Part model, mm, in its own coordinate system. A direction names the side the tool comes from. Round coordinates to 2 decimals unless told otherwise and drop trailing zeros.
```python
from build123d import *

# Parameters (mm, degrees)
SKETCH1_R           = 42.5
BOSS_EXTRUDE1_DEPTH = 115
SKETCH2_R           = 41
CUT_EXTRUDE3_DEPTH  = 115
SKETCH9_W           = 4.5
SKETCH9_H           = 9
CUT_EXTRUDE5_DEPTH  = 115
SKETCH14_W          = 4
SKETCH14_H          = 2.5
CUT_EXTRUDE8_DEPTH  = 115
SKETCH16_W          = 8
SKETCH16_H          = 4.5
CUT_EXTRUDE9_DEPTH  = 115
BOSS_EXTRUDE2_START = 1
SKETCH19_R          = 41
BOSS_EXTRUDE2_DEPTH = 1
SKETCH21_R          = 3
BOSS_EXTRUDE3_DEPTH = 50
SHELL1_T            = -0.3
SKETCH24_R          = 3
BOSS_EXTRUDE4_DEPTH = 35
SHELL2_START        = 19
SHELL2_OUTLINE_R    = 2.7
SHELL2_DEPTH        = 35
SKETCH25_R          = 3
BOSS_EXTRUDE5_DEPTH = 45
SHELL5_T            = -0.03
SKETCH26_W          = 30
SKETCH26_H          = 15
BOSS_EXTRUDE6_DEPTH = 5


# Read off the part's stored shape, not the designer's step: Shell2
with BuildPart() as part:
    # Sketch1 → Boss-Extrude1 (new body)
    with BuildSketch(Plane(origin=(0, 0, 0), x_dir=(1, 0, 0), z_dir=(0, 1, 0))):
        with Locations(Location((0, 0, 0), (0, 0, 270))):
            Circle(SKETCH1_R)
    extrude(amount=BOSS_EXTRUDE1_DEPTH)

    # Sketch7 → Loft2 section 0
    with BuildSketch(Plane.XZ):
        with BuildLine():
            Line((-15.1377027, -38.271634302), (14.891561193, -38.271634302))
            Line((14.891561193, -38.271634302), (14.891561193, -51.96970786))
            Line((14.891561193, -51.96970786), (-15.1377027, -51.96970786))
            Line((-15.1377027, -51.96970786), (-15.1377027, -38.271634302))
        make_face()
    # Sketch6 → Loft2 section 1
    with BuildSketch(Plane(origin=(0, 115, 0), x_dir=(1, 0, 0), z_dir=(0, 1, 0))):
        with BuildLine():
            Line((-10.741203576, 39.96970786), (9.258796424, 39.96970786))
            Line((9.258796424, 39.96970786), (9.258796424, 51.96970786))
            Line((9.258796424, 51.96970786), (-10.741203576, 51.96970786))
            Line((-10.741203576, 51.96970786), (-10.741203576, 39.96970786))
        make_face()
    loft()

    # Sketch2 → Cut-Extrude3 (cut)
    with BuildSketch(Plane(origin=(0, 115, 0), x_dir=(1, 0, 0), z_dir=(0, 1, 0))):
        with Locations(Location((0, 0, 0), (0, 0, 270))):
            Circle(SKETCH2_R)
    extrude(amount=-CUT_EXTRUDE3_DEPTH, mode=Mode.SUBTRACT)

    # Sketch9 → Cut-Extrude5 (cut)
    with BuildSketch(Plane(origin=(0, 115, 0), x_dir=(1, 0, 0), z_dir=(0, 1, 0))):
        with Locations((-6.991203576, 47.46970786)):
            Rectangle(SKETCH9_W, SKETCH9_H)
        with Locations((5.508796424, 47.46970786)):
            Rectangle(SKETCH9_W, SKETCH9_H)
    extrude(amount=-CUT_EXTRUDE5_DEPTH, mode=Mode.SUBTRACT)

    # Sketch14 → Cut-Extrude8 (cut)
    with BuildSketch(Plane(origin=(0, 115, 0), x_dir=(1, 0, 0), z_dir=(0, 1, 0))):
        with Locations((-0.741203576, 44.290749204)):
            Rectangle(SKETCH14_W, SKETCH14_H)
    extrude(amount=-CUT_EXTRUDE8_DEPTH, mode=Mode.SUBTRACT)

    # Sketch16 → Cut-Extrude9 (cut)
    with BuildSketch(Plane(origin=(0, 115, 0), x_dir=(1, 0, 0), z_dir=(0, 1, 0))):
        with Locations((-0.741203576, 49.71970786)):
            Rectangle(SKETCH16_W, SKETCH16_H)
    extrude(amount=-CUT_EXTRUDE9_DEPTH, mode=Mode.SUBTRACT)

    # Sketch19 → Boss-Extrude2 (add)
    with BuildSketch(Plane(origin=(0, 54, 0), x_dir=(1, 0, 0), z_dir=(0, 1, 0)).offset(BOSS_EXTRUDE2_START)):
        with Locations(Location((0, 0, 0), (0, 0, 270))):
            Circle(SKETCH19_R)
    extrude(amount=-BOSS_EXTRUDE2_DEPTH)

    # Sketch21 → Boss-Extrude3 (add)
    with BuildSketch(Plane.XZ.offset(-54)):
        with Locations(Location((-35.3, 0, 0), (0, 0, 90))):
            Circle(SKETCH21_R)
        with Locations(Location((35.3, 0, 0), (0, 0, 90))):
            Circle(SKETCH21_R)
    extrude(amount=BOSS_EXTRUDE3_DEPTH)

    # Shell1
    shell1_openings = [part.faces().sort_by_distance(p)[0] for p in [
        (-35.3, 4, 0),
        (35.3, 4, 0),
    ]]
    offset(amount=SHELL1_T, openings=shell1_openings, kind=Kind.INTERSECTION)

    # Sketch24 → Boss-Extrude4 (add)
    with BuildSketch(Plane.XZ.offset(-54)):
        with Locations(Location((7.5, 30, 0), (0, 0, 90))):
            Circle(SKETCH24_R)
        with Locations(Location((-7.5, 30, 0), (0, 0, 90))):
            Circle(SKETCH24_R)
    extrude(amount=BOSS_EXTRUDE4_DEPTH)

    # Shell2 outline → Shell2 (cut)
    with BuildSketch(Plane(origin=(0, 0, 0), x_dir=(1, 0, 0), z_dir=(0, 1, 0)).offset(SHELL2_START)):
        with Locations((-7.5, -30)):
            Circle(SHELL2_OUTLINE_R)
        with Locations((7.5, -30)):
            Circle(SHELL2_OUTLINE_R)
    extrude(amount=SHELL2_DEPTH, mode=Mode.SUBTRACT)

    # Sketch25 → Boss-Extrude5 (add)
    with BuildSketch(Plane.XZ.offset(-54)):
        with Locations(Location((14, -32.5, 0), (0, 0, 90))):
            Circle(SKETCH25_R)
        with Locations(Location((-14, -32.5, 0), (0, 0, 90))):
            Circle(SKETCH25_R)
    extrude(amount=BOSS_EXTRUDE5_DEPTH)

    # Shell5
    shell5_openings = [part.faces().sort_by_distance(p)[0] for p in [
        (-14, 9, -32.5),
        (14, 9, -32.5),
    ]]
    offset(amount=SHELL5_T, openings=shell5_openings, kind=Kind.INTERSECTION)

    # Sketch26 → Boss-Extrude6 (add)
    with BuildSketch(Plane.XZ.offset(-54)):
        Rectangle(SKETCH26_W, SKETCH26_H)
    extrude(amount=BOSS_EXTRUDE6_DEPTH)


solid = part.part
```
Q1. Drop flat-ended pins along their axis: pin 1 (0.8 mm diameter, centred on y = 63, z = -44, fed in from -X); pin 2 (5 mm diameter, centred on y = 87, z = 6, fed in from -X); pin 3 (6 mm diameter, centred on y = 50.5, z = -12.5, fed in from +X); pin 4 (12 mm diameter, centred on x = 5.5, z = -41.5, fed in from -Y). Give the stop position or say it passes through.
Values follow:
pin 1: stops at x = -12.74
pin 2: stops at x = -42.36
pin 3: stops at x = 41.42
pin 4: stops at y = 0
Q2. Which spindle directions (+Z, -Z, +X, -X, +Y, -Y) get a long thin tool onto all of the face, cutting with end or side? Do faces 1 (the flat face through (1, 54.03, -1)), 2 (the flat face through (0, 52, -7.5)). Say none if no direction does.
Values follow:
face 1: none
face 2: -Y
Q3. Cut at A-A on z = 0. State how many separate pieces and enclosed holes the cut face has, plus the area to 3 significant figures.
Values follow:
separate pieces: 2
enclosed holes: 2
area: 199 mm2
